Geometry check sheet. Reference: the model listing, model coordinates, mm. A direction names the side the tool comes from. Give positions to 0.01 mm unless a question says otherwise; leave off trailing zeros. Order: outer loops, then holes, each group sorted by start corner. A loop starts at its lowest first (then second) coordinate and runs counter-clockwise, first axis right, second up. Notation, with made-up numbers: M 49.25,37.25 L 72.25,37.25 A19 ccw 72.25,74.25 Z; hole C 53.25,4 d6. An arc over 180 degrees is marked long. Answer as CSV lines item,"result". Start each with the question number.
```python
from build123d import *

# Parameters (mm, degrees)
EXTRUDE_1_DEPTH     = 6
SKETCH_7_R          = 1.5
CUT_EXTRUDE_3_DEPTH = 31
CUT_EXTRUDE_START   = -2.6
SKETCH_8_R          = 10.5
CUT_EXTRUDE_4_DEPTH = 2.6
SKETCH_9_R          = 0.75
CUT_EXTRUDE_5_DEPTH = 10
SKETCH_10_R         = 4.5
CUT_EXTRUDE_6_DEPTH = 10


with BuildPart() as part:
    # 草图2 → 凸台-拉伸1 (new body)
    with BuildSketch(Plane.XY):
        with BuildLine():
            Line((-5.050750258, -65.386258364), (17.949249742, -65.386258364))
            ThreePointArc((17.949249742, -65.386258364), (23.949249742, -71.386258364), (17.949249742, -77.386258364))
            Line((17.949249742, -77.386258364), (-5.050750258, -77.386258364))
            ThreePointArc((-5.050750258, -77.386258364), (-23.050750258, -71.386258364), (-5.050750258, -65.386258364))
        make_face()
    extrude(amount=-EXTRUDE_1_DEPTH)

    # 草图7 → 切除-拉伸3 (cut)
    with BuildSketch(Plane.XY):
        with Locations((17.949249742, -71.386258364)):
            Circle(SKETCH_7_R)
    extrude(amount=-CUT_EXTRUDE_3_DEPTH, mode=Mode.SUBTRACT)

    # 草图8 → 切除-拉伸4 (cut)
    with BuildSketch(Plane(origin=(0, 0, -6), x_dir=(-1, 0, 0), z_dir=(0, 0, -1)).offset(CUT_EXTRUDE_START)):
        with Locations((13.050750258, -71.386258364)):
            Circle(SKETCH_8_R)
    extrude(amount=CUT_EXTRUDE_4_DEPTH, mode=Mode.SUBTRACT)

    # 草图9 → 切除-拉伸5 (cut)
    with BuildSketch(Plane(origin=(0, 0, -3.4), x_dir=(-1, 0, 0), z_dir=(0, 0, -1))):
        with Locations(Location((6.050750258, -71.386258364, 0), (0, 0, 90))):
            Circle(SKETCH_9_R)
        with Locations(Location((6.050750258, -74.386258364, 0), (0, 0, 90))):
            Circle(SKETCH_9_R)
        with Locations(Location((6.050750258, -68.386258364, 0), (0, 0, 90))):
            Circle(SKETCH_9_R)
        with Locations(Location((10.050750258, -78.386258364, 0), (0, 0, 90))):
            Circle(SKETCH_9_R)
        with Locations(Location((13.050750258, -78.386258364, 0), (0, 0, 90))):
            Circle(SKETCH_9_R)
        with Locations(Location((16.050750258, -78.386258364, 0), (0, 0, 90))):
            Circle(SKETCH_9_R)
        with Locations(Location((20.050750258, -74.386258364, 0), (0, 0, 90))):
            Circle(SKETCH_9_R)
        with Locations(Location((20.050750258, -71.386258364, 0), (0, 0, 90))):
            Circle(SKETCH_9_R)
        with Locations(Location((20.050750258, -68.386258364, 0), (0, 0, 90))):
            Circle(SKETCH_9_R)
        with Locations(Location((16.050750258, -64.386258364, 0), (0, 0, 90))):
            Circle(SKETCH_9_R)
        with Locations(Location((13.050750258, -64.386258364, 0), (0, 0, 90))):
            Circle(SKETCH_9_R)
        with Locations(Location((10.050750258, -64.386258364, 0), (0, 0, 90))):
            Circle(SKETCH_9_R)
    extrude(amount=-CUT_EXTRUDE_5_DEPTH, mode=Mode.SUBTRACT)

    # 草图10 → 切除-拉伸6 (cut)
    with BuildSketch(Plane(origin=(0, 0, -3.4), x_dir=(-1, 0, 0), z_dir=(0, 0, -1))):
        with Locations(Location((13.050750258, -71.386258364, 0), (0, 0, 90))):
            Circle(SKETCH_10_R)
    extrude(amount=-CUT_EXTRUDE_6_DEPTH, mode=Mode.SUBTRACT)


solid = part.part
```
Item 1: Scan lines: line 1 along X through (y, z) = (-71, -1.7); line 2 along X through (y, z) = (-71.25, -5); line 3 along Y through (x, z) = (5.5, -1.4). Record each from-to range of solid material in increasing order.
Item 2: Draft check along Y on faces 1 (the face through (-16.338, -77.693, -1.724)), 2 (the face through (1, -71, 0)), 3 (the face through (18.64, -72.72, -2.96)), 4 (the face through (-23.045, -71.736, -1.676)). Enter one of: pulls with the +Y half, pulls with the -Y half, needs draft (parallel to the pull), parting line crosses it, or undercut.
Item 3: Depth check by flat-ended pin: pin 1 Ø1.8 at (x, z) = (1, -4) entering from -Y; pin 2 Ø1.4 at (x, y) = (-13.05, -78.39) entering from +Z; pin 3 Ø1.5 at (y, z) = (-66.5, -4) entering from -X; pin 4 Ø2.5 at (x, y) = (-6.05, -68.39) entering from -Z. Enter the tip coordinate at first touch or a pass-through.
Item 4: Section check B-B on z = -0.65. Give the number of separate pieces and of enclosed holes in the cut face, then the cut area to 3 significant figures.
Item 5: Section check C-C on x = 11.5. Record the boundary of the cut face in (y, z), then the cut area to 3 significant figures.
Item 6: Section check D-D on x = -8. Record the boundary of the cut face in (y, z), then the cut area to 3 significant figures.
Item 7: Section check A-A on y = -64.5. Record the boundary of the cut face in (x, z).
Item 8: Access from +Z, -Z, +X, -X, +Y, -Y to the whole of each face (thin tool, end or side, straight path). Record for faces 5 (the face through (-13.338, -77.693, -1.724)), 6 (the face through (6, -65.386, -3)), 7 (the face through (7, -77.386, -3)), 8 (the face through (-2.55, -71.3, -4.68)).
Numbers:
1,line 1,"-23.04 to -20.69, -19.41 to -17.53, -8.57 to -6.69, -5.41 to 16.5, 19.4 to 23.94"
1,line 2,"-2.55 to 16.46, 19.44 to 23.95"
1,line 3,"-77.39 to -65.39"
2,face 1,"undercut"
2,face 2,"needs draft"
2,face 3,"undercut"
2,face 4,"parting line crosses it"
3,pin 1,"y = -77.39"
3,pin 2,"through"
3,pin 3,"x = -22.01"
3,pin 4,"z = -3.4"
4,separate pieces,"1"
4,enclosed holes,"14"
4,area,"538 mm2"
5,outline,"M -77.39,-6 L -65.39,-6 L -65.39,0 L -77.39,0 Z"
5,area,"72.0 mm2"
6,outline,"M -80.02,-3.4 L -62.76,-3.4 L -62.76,0 L -80.02,0 Z"
6,area,"58.7 mm2"
7,outline,"M -20.3,-3.4 L -16.79,-3.4 L -16.79,0 L -20.3,0 Z; M -15.31,-3.4 L -13.79,-3.4 L -13.79,0 L -15.31,0 Z; M -12.31,-3.4 L -10.79,-3.4 L -10.79,0 L -12.31,0 Z; M -9.31,-3.4 L -5.8,-3.4 L -5.8,0 L -9.31,0 Z"
8,face 5,"+Z, -Z"
8,face 6,"+Z, -Z, +X, +Y"
8,face 7,"+Z, -Z, +X, -Y"
8,face 8,"-Z, -X"
